```python
from build123d import *

# Parameters (mm, degrees)
F0_R     = 12
F0_R_2   = 2.05
F1_DEPTH = 6.8
F2_DEPTH = 0.5
F3_SIZE  = 0.5
F4_SIZE  = 6


with BuildPart() as f1:
    # F0 (on Top) → F1 (new body)
    with BuildSketch(Plane.XY):
        Circle(F0_R)
        Circle(F0_R_2, mode=Mode.SUBTRACT)
    extrude(amount=F1_DEPTH)

    # F0 (on Top) → F2 (join)
    with BuildSketch(Plane.XY):
        Circle(F0_R_2)
    extrude(amount=F2_DEPTH)

    # F3
    f3_edges = [f1.edges().sort_by_distance(p)[0] for p in [
        (-2.05, 0, 6.8),
    ]]
    chamfer(f3_edges, length=F3_SIZE)

    # F4
    f4_edges = [f1.edges().sort_by_distance(p)[0] for p in [
        (-12, 0, 6.8),
    ]]
    chamfer(f4_edges, length=F4_SIZE)


solid = f1.part
```
Geometry check sheet. Reference: the model listing, model coordinates, mm. A direction names the side the tool comes from. Give positions to 0.01 mm unless a question says otherwise; leave off trailing zeros. Order: outer loops, then holes, each group sorted by start corner. A loop starts at its lowest first (then second) coordinate and runs counter-clockwise, first axis right, second up. Notation, with made-up numbers: (25.25, -27) - (62.25, -27) arc R5 ccw to (62.25, -23) - close; hole circle Ø2 at (33, 45.5). An arc over 180 degrees is marked (long way). Write item = value, one per line. Start each with the question number.
1) Section check B-B (z = 2.5). Enter the section's corners in (x, y).
2) Draft check along X on faces 1 (the cylindrical face through (-11.99, 0.53, 0.39)), 2 (the flat face through (0, 0, 0.5)), 3 (the flat face through (3, 0, 6.8)). Enter one of: released by +X, released by -X, zero draft, split by the parting line, or undercut.
3) Scan lines: L1, parallel to Y at x = 0, z = 3.45; L2, parallel to Y at x = 1.75, z = 2; L3, parallel to X at y = -0.5, z = 6.5. Record each from-to range of solid material in increasing order.
4) Section check D-D (z = 4.75). Enter the section's corners in (x, y).
5) Access from +Z, -Z, +X, -X, +Y, -Y to the whole of each face (thin tool, end or side, straight path). Record for faces 4 (the flat face through (0, 0, 0)), 5 (the cylindrical face through (-0.267, 2.033, 3.359)).
6) Gauge pin test, flat ends, axial feed: pin 1 Ø3 at (y, z) = (5.5, 5.5) entering from -X; pin 2 Ø1 at (x, z) = (5, 6) entering from +Y; pin 3 Ø1 at (y, z) = (2.5, 4.5) entering from -X. Record the tip position at first contact, or that the pin passes through.
7) Section check A-A (x = 0). Enter the section's corners in (y, z).
Geometry check:
q1.outline = circle Ø20.6 at (0, 0); hole circle Ø4.1 at (0, 0)
q2.face_1 = split by the parting line
q2.face_2 = undercut
q2.face_3 = zero draft
q3.L1 = -9.35 to -2.05, 2.05 to 9.35
q3.L2 = -10.66 to -1.07, 1.07 to 10.66
q3.L3 = -6.28 to -2.19, 2.19 to 6.28
q4.outline = circle Ø16.1 at (0, 0); hole circle Ø4.1 at (0, 0)
q5.face_4 = -Z, +X, -X, +Y, -Y
q5.face_5 = +Z
q6.pin_1 = -7.17
q6.pin_2 = 5.46
q6.pin_3 = -8.46
q7.outline = (-12, 0) - (12, 0) - (12, 0.8) - (6, 6.8) - (2.55, 6.8) - (2.05, 6.3) - (2.05, 0.5) - (-2.05, 0.5) - (-2.05, 6.3) - (-2.55, 6.8) - (-6, 6.8) - (-12, 0.8) - close
